Drawing for the job (mm, zero at the part's lowest x, y, z). Round coordinates to 2 decimals unless told otherwise and drop trailing zeros. Loops run counter-clockwise (first coordinate to the right, second up) from the corner with the lowest first, then second, coordinate; pieces in that order, holes last. Notation, with made-up numbers: M 37.5,4 L 69.5,4 A24 cw 69.5,38 Z; hole C -23.75,40.5 d2. An arc over 180 degrees is marked long. Use a Markdown table: item, result. Add a question column.
Q1. Probe line 1 (Z direction, x = 25, y = 10.75); line 2 (X direction, y = 13.5, z = 47); line 3 (X direction, y = 3.75, z = 21.5). List the from-to ranges inside material, lowest first. Write a range as from..to.
Q2. Mould opens along Z. For the marked faces 1 and 2 say: +Z half, -Z half, draft (parallel to the pull), parting line (faces both ways), or undercut.
Q3. Pin check, flat tip, straight feed: pin 1 (1.5 mm diameter, centred on x = 171.5, z = 11, fed in from +Y). Stop position of the tip, or through.
Q4. Cut at B-B (z = 17.5). Give the cut face in (x, y).
Q5. Cut at D-D (z = 45.5). Give the cut face in (x, y).
Q6. Cut at C-C (x = 192). Give the cut face in (y, z), plus the area to 3 significant figures.
Q7. Cut at A-A (y = 12.25). Give the cut face in (x, z), plus the area to 3 significant figures.
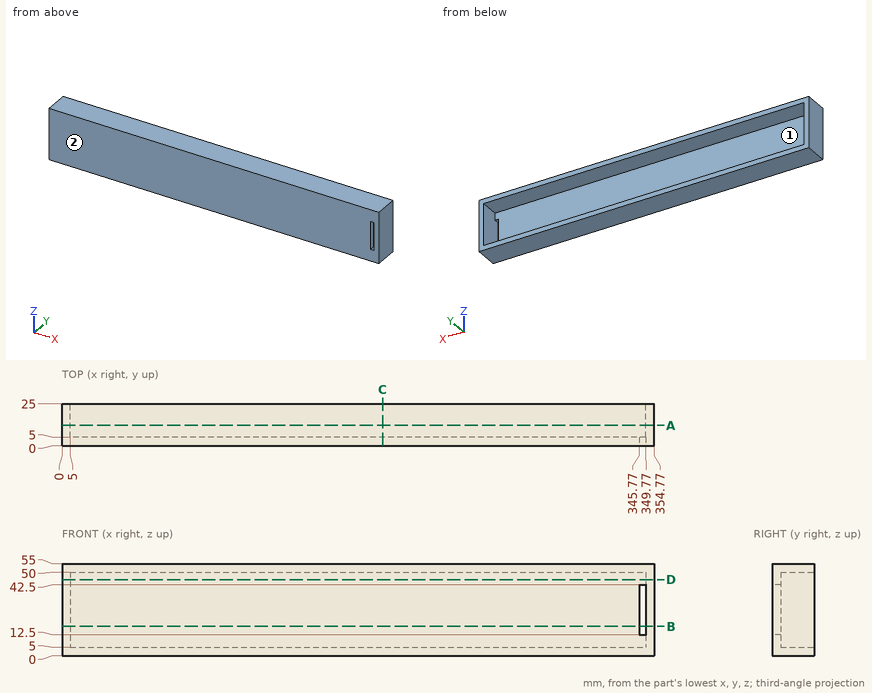
Checked values:
| question | item | result |
|---|---|---|
| 1 | line 1 | z = 0..5, 50..55 |
| 1 | line 2 | x = 0..5, 349.77..354.77 |
| 1 | line 3 | x = 0..345.77, 349.77..354.77 |
| 2 | face 1 | undercut |
| 2 | face 2 | draft |
| 3 | pin 1 | stops at y = 5 |
| 4 | outline | M 0,0 L 345.77,0 L 345.77,5 L 5,5 L 5,25 L 0,25 Z; M 349.77,0 L 354.77,0 L 354.77,25 L 349.77,25 Z |
| 5 | outline | M 0,0 L 354.77,0 L 354.77,25 L 349.77,25 L 349.77,5 L 5,5 L 5,25 L 0,25 Z |
| 6 | outline | M 0,0 L 25,0 L 25,5 L 5,5 L 5,50 L 25,50 L 25,55 L 0,55 Z |
| 6 | area | 475 mm^2 |
| 7 | outline | M 0,0 L 354.77,0 L 354.77,55 L 0,55 Z; hole M 5,5 L 349.77,5 L 349.77,50 L 5,50 Z |
| 7 | area | 4,000 mm^2 |
